Check sheet for the modelled part. Datum: model origin and axes. Units: mm. Round coordinates to 2 decimals unless told otherwise and drop trailing zeros. Write each loop counter-clockwise with the first axis right and the second up, starting at its lowest first coordinate (ties: lowest second). Pieces come first, ordered by that corner, then holes. Notation, with made-up numbers: (17, 41) -> (37, 41) arc R14 cw to (37, 53) -> close; hole circle Ø10 at (7, 72.25). An arc over 180 degrees is marked (long way). One line per item, written item: value.
Autodesk Inventor part; units mm, degrees
ref_plane "YZ Plane" through (0, 0, 0) normal (1, 0, 0) x (0, 1, 0)
ref_plane "XZ Plane" through (0, 0, 0) normal (0, 1, 0) x (-1, 0, 0)
ref_plane "XY Plane" through (0, 0, 0) normal (0, 0, 1) x (1, 0, 0)
sketch "Sketch1" plane through (0, 0, 0) normal (0, 0, 1) x (1, 0, 0)
  line L0 (-60, 30) -> (60, 30)
  line L1 (60, 30) -> (60, -30)
  line L2 (60, -30) -> (-60, -30)
  line L3 (-60, -30) -> (-60, 30)
  line L4 (-60, 30) -> (60, -30) construction
  line L5 (60, 30) -> (-60, -30) construction
  line L6 (-60, 24) -> (60, 24) construction
  line L7 (60, 24) -> (60, -24) construction
  line L8 (60, -24) -> (-60, -24) construction
  line L9 (-60, -24) -> (-60, 24) construction
  line L10 (-60, 24) -> (60, -24) construction
  line L11 (60, 24) -> (-60, -24) construction
  line L12 (-59.6915, 27) -> (60.3085, 27) construction
  line L13 (59.9134, -27) -> (-60.0866, -27) construction
  line L14 (-55, 34.9894) -> (-55, -41.0431) construction
  line L15 (55, 34.9894) -> (55, -41.0431) construction
  line L16 (-0.0866, 42.6852) -> (-0.0866, -44.8416)
  line L17 (-70.7157, 0) -> (86.0605, 0)
  line L18 (-55.95, 29.5) -> (-54.05, 29.5)
  line L19 (-54.05, 29.5) -> (-54.05, 24.5)
  line L20 (-54.05, 24.5) -> (-55.95, 24.5)
  line L21 (-55.95, 24.5) -> (-55.95, 29.5)
  line L22 (-55.95, 29.5) -> (-54.05, 24.5) construction
  line L23 (-54.05, 29.5) -> (-55.95, 24.5) construction
  line L24 (55.7768, 29.5) -> (53.8768, 29.5)
  line L25 (53.8768, 29.5) -> (53.8768, 24.5)
  line L26 (53.8768, 24.5) -> (55.7768, 24.5)
  line L27 (55.7768, 24.5) -> (55.7768, 29.5)
  line L28 (55.7768, 29.5) -> (53.8768, 24.5) construction
  line L29 (53.8768, 29.5) -> (55.7768, 24.5) construction
  line L30 (-55.95, -29.5) -> (-54.05, -29.5)
  line L31 (-54.05, -29.5) -> (-54.05, -24.5)
  line L32 (-54.05, -24.5) -> (-55.95, -24.5)
  line L33 (-55.95, -24.5) -> (-55.95, -29.5)
  line L34 (-55.95, -29.5) -> (-54.05, -24.5) construction
  line L35 (-54.05, -29.5) -> (-55.95, -24.5) construction
  line L36 (53.8768, -29.5) -> (53.8768, -24.5)
  line L37 (53.8768, -24.5) -> (55.7768, -24.5)
  line L38 (55.7768, -24.5) -> (55.7768, -29.5)
  line L39 (55.7768, -29.5) -> (53.8768, -24.5) construction
  line L40 (53.8768, -29.5) -> (55.7768, -24.5) construction
  line L41 (55.7768, -29.5) -> (53.8768, -29.5)
  point P0 (0, 0)
  point P1 (-55, 27)
  point P2 (54.8268, 27)
  point P3 (-55, -27)
  point P4 (54.8268, -27)
  dimension "d0" = 120
  dimension "d1" = 60
  dimension "d5" = 48
  dimension "d6" = 6
  dimension "d7" = 3
  dimension "d9" = 3
  dimension "d10" = 5
  dimension "d11" = 5
  dimension "d26" = 1.9
  dimension "d27" = 5
extrude "Extrusion1" add sketch "Sketch1" along normal blind 4 contours L0 L16 L17 L3 | L0 L1 L17 L16 | L17 L16 L2 L3 | L17 L1 L2 L16 | L18 L19 L20 L21 | L27 L26 L25 L24 | L33 L32 L31 L30 | L36 L37 L38 L41
sketch "Sketch2" plane through (60, -30, 0) normal (1, 0, 0) x (0, 0, -1)
  line L0 (-8.9857, 57) -> (8.9833, 57) construction
  line L1 (0, 60) -> (-4, 60)
  line L2 (-2, 63.5324) -> (-2, -21.5348) construction
  line L3 (0, 60) -> (0, 0) construction
  line L4 (-7.253, 3) -> (5.1126, 3) construction
  line L5 (0, 0) -> (-4, 0) construction
  circle A0 centre (-2, 57) radius 1.25
  circle A1 centre (-2, 3) radius 1.25
  point P0 (0, 30)
  dimension "d12" = 3
  dimension "d13" = 2
  dimension "d14" = 3
  dimension "d15" = 2.5
  dimension "d16" = 2.5
extrude "Extrusion2" cut sketch "Sketch2" against normal blind 20
sketch "Sketch3" plane through (-60, -30, 0) normal (-1, 0, 0) x (0, 0, 1)
  line L0 (-7.4279, 57) -> (13.0105, 57) construction
  line L1 (2, 62.779) -> (2, -22.3608) construction
  line L2 (-5.3723, 3) -> (8.7736, 3) construction
  line L3 (0, 60) -> (4, 60) construction
  line L4 (0, 0) -> (4, 0) construction
  line L5 (0, 0) -> (0, 60) construction
  circle A0 centre (2, 57) radius 1.25
  circle A1 centre (2, 3) radius 1.25
  point P0 (0, 30)
  dimension "d19" = 3
  dimension "d20" = 3
  dimension "d21" = 2
  dimension "d22" = 2.5
  dimension "d23" = 2.5
extrude "Extrusion3" cut sketch "Sketch3" against normal blind 20
extrude "Extrusion4" cut sketch "Sketch1" along normal blind 10 contours L18 L19 L20 L21 | L27 L26 L25 L24 | L33 L32 L31 L30 | L36 L37 L38 L41
sketch "Sketch5" plane through (0, 0, 0) normal (0, 0, -1) x (-1, 0, 0)
  line L0 (-55, 28) -> (30, 28) construction
  line L1 (30, 28) -> (30, -28) construction
  line L2 (30, -28) -> (-55, -28) construction
  line L3 (-55, -28) -> (-55, 28) construction
  line L4 (60, 30) -> (-60, 30)
  line L5 (-60, -30) -> (60, -30)
  line L6 (-60, 30) -> (-60, -30)
  line L7 (-61.4504, 24.5) -> (34.2975, 24.5) construction
  line L8 (-31.5, 29.0313) -> (-31.5, -33.267) construction
  line L9 (26.5, 28.5391) -> (26.5, -33.7592) construction
  line L10 (-62.9373, -24.5) -> (32.8105, -24.5) construction
  circle A0 centre (-31.5, 24.5) radius 3.1
  circle A1 centre (26.5, 24.5) radius 3.1
  circle A2 centre (-31.5, -24.5) radius 3.1
  circle A3 centre (26.5, -24.5) radius 3.1
  circle A4 centre (-31.5, 24.5) radius 0.85
  circle A5 centre (26.5, 24.5) radius 0.85
  circle A6 centre (-31.5, -24.5) radius 0.85
  circle A7 centre (26.5, -24.5) radius 0.85
  point P0 (0, 0)
  dimension "d32" = 2
  dimension "d35" = 56
  dimension "d36" = 60
  dimension "d37" = 85
  dimension "d38" = 5
  dimension "d39" = 3.5
  dimension "d40" = 3.5
  dimension "d41" = 3.5
  dimension "d42" = 58
  dimension "d43" = 6.2
  dimension "d44" = 6.2
  dimension "d45" = 6.2
  dimension "d46" = 6.2
  dimension "d47" = 1.7
  dimension "d48" = 1.7
  dimension "d49" = 1.7
  dimension "d50" = 1.7
extrude "Extrusion6" add sketch "Sketch5" along normal blind 3
extrude "Extrusion8" cut sketch "Sketch5" against normal blind 5 contours A4 | A5 | A6 | A7
sketch "Sketch6" plane through (0, 0, 4) normal (0, 0, 1) x (1, 0, 0)
  line L0 (55, -26.7) -> (-13.6, -26.7) construction
  line L1 (-13.6, -26.7) -> (-13.6, 26.6) construction
  line L2 (-13.6, 26.6) -> (55, 26.6) construction
  line L3 (55, 26.6) -> (55, -26.7) construction
  line L4 (60, -30) -> (60, 30)
  line L5 (-60, -30) -> (60, -30)
  line L6 (60, 30) -> (-60, 30)
  line L7 (-11.1, 28.3746) -> (-11.1, -43.0952) construction
  line L8 (41, 27.7316) -> (41, -43.7382) construction
  line L9 (39.7, 28.5262) -> (39.7, -42.9435) construction
  line L10 (-16.1238, 24.1) -> (57.2628, 24.1) construction
  line L11 (-13.8231, 19) -> (59.5635, 19) construction
  line L12 (-15.4929, -8.9) -> (57.8937, -8.9) construction
  line L13 (-14.4245, -24.2) -> (58.9621, -24.2) construction
  circle A0 centre (-11.1, 19) radius 0.5
  circle A1 centre (-11.1, -8.9) radius 0.5
  circle A2 centre (41, 24.1) radius 0.5
  circle A3 centre (39.7, -24.2) radius 0.5
  point P0 (0, 0)
  dimension "d57" = 53.3
  dimension "d58" = 68.6
  dimension "d59" = 5
  dimension "d60" = 3.3
  dimension "d61" = 3.4
  dimension "d62" = 2.5
  dimension "d63" = 2.5
  dimension "d64" = 14
  dimension "d65" = 1.3
  dimension "d66" = 50.8
  dimension "d68" = 27.9
  dimension "d69" = 5.1
  dimension "d70" = 35.5
  dimension "d71" = 1
  dimension "d72" = 1
  dimension "d73" = 1
  dimension "d74" = 1
extrude "Extrusion9" cut sketch "Sketch6" against normal blind 5
properties part number "Boardcarrier"
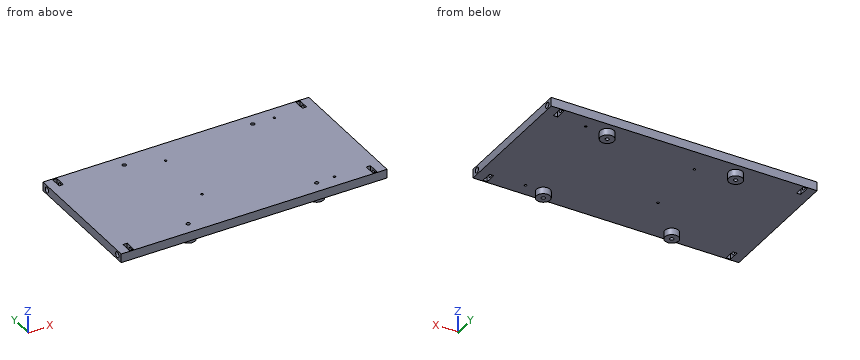
Item 1: Sectioned sample at B-B (y = -0.5). Enter the section's corners in (x, z).
Result set:
outline: (-60, 0) -> (60, 0) -> (60, 4) -> (-60, 4) -> close
Item 2: Depth check by flat-ended pin: pin 1 (8 mm diameter, centred on x = 46, y = -8, fed in from -Z); pin 2 (2 mm diameter, centred on y = 27, z = 2, fed in from -X). Enter the tip coordinate at first touch or a pass-through.
Result set:
pin 1: z = 0
pin 2: x = -40
Item 3: Material ranges on line 1 along Y through (x, z) = (-57.1, 2); line 2 along Y through (x, z) = (-26.5, 1.25); line 3 along Z through (x, y) = (-49, -24), recorded low to high.
Result set:
line 1: -30 to -28.25, -25.75 to 25.75, 28.25 to 30
line 2: -30 to -25.35, -23.65 to 23.65, 25.35 to 30
line 3: 0 to 4
Item 4: Sectioned sample at C-C (x = -33). Enter the section's corners in (y, z), then the cut area to 3 significant figures.
Result set:
outline: (-30, 0) -> (30, 0) -> (30, 4) -> (-30, 4) -> close
area: 240 mm^2
Item 5: Sectioned sample at A-A (x = -51.5). Enter the section's corners in (y, z).
Result set:
outline: (-30, 0) -> (30, 0) -> (30, 4) -> (-30, 4) -> close; hole circle Ø2.5 at (-27, 2); hole circle Ø2.5 at (27, 2)
